Solid Edge part; units mm, degrees
sketch "Sketch1" plane through (0, 0, 0) normal (0, -1, 0) x (1, 0, 0)
  line L0 (0, 120) -> (0, 0)
  line L1 (0, 0) -> (100, 0)
  line L2 (100, 0) -> (100, 120)
  line L3 (100, 120) -> (0, 120)
extrude "Protrusion1" add sketch "Sketch1" against normal blind 150
hole "Hole1" at (25, 25, 120) direction (0, 0, -1) diameter 8.376 depth 35 start chamfer 1 start chamfer angle 45
hole "Hole2" at (25, 125, 120) direction (0, 0, -1) diameter 8.376 depth 35 start chamfer 1 start chamfer angle 45
hole "Hole3" at (75, 125, 120) direction (0, 0, -1) diameter 8.376 depth 35 start chamfer 1 start chamfer angle 45
hole "Hole4" at (75, 25, 120) direction (0, 0, -1) diameter 8.376 depth 35 start chamfer 1 start chamfer angle 45
hole "Hole5" at (25, 25, 0) direction (0, 0, 1) diameter 8.376 depth 35 start chamfer 1 start chamfer angle 45
hole "Hole6" at (75, 25, 0) direction (0, 0, 1) diameter 8.376 depth 35 start chamfer 1 start chamfer angle 45
hole "Hole7" at (75, 125, 0) direction (0, 0, 1) diameter 8.376 depth 35 start chamfer 1 start chamfer angle 45
hole "Hole8" at (25, 125, 0) direction (0, 0, 1) diameter 8.376 depth 35 start chamfer 1 start chamfer angle 45
hole "Achsenhalterung_Schubkarr" at (0, 75, 60) direction (1, 0, 0) diameter 20 end through all start chamfer 1 start chamfer angle 45 end chamfer 1 end chamfer angle 45
Design review of the part built by this model. Coordinates are the model's own, in mm. A direction names the side the tool comes from. Coordinates: 2 decimals unless noted, no trailing zeros. Order: outer loops, then holes, each group sorted by start corner. A loop starts at its lowest first (then second) coordinate and runs counter-clockwise, first axis right, second up.
Item 1: For line 1 (Y direction, x = 75, z = 12); line 2 (X direction, y = 25, z = 15.5); line 3 (Y direction, x = 57, z = 60), list the stretches that pass through material, from the lowest coordinate up.
Item 2: Take a section at D-D, the plane x = 87. Write out the cut boundary in (y, z).
Item 3: For pin 1 Ø4 at (x, y) = (23, 126) entering from -Z; pin 2 Ø2.5 at (x, y) = (76, 24) entering from +Z; pin 3 Ø4 at (x, y) = (26.5, 23) entering from +Z, all flat-tipped, find the tip position at first contact; note any pin that passes through.
Item 4: The part is to be moulded in two halves that separate along Y. For faces 1 (the flat face through (0, 74, 74)), 2 (the flat face through (75, 25, 85)), 3 (the flat face through (51, 0, 61)), say which applies: pulls with the +Y half, pulls with the -Y half, needs draft (parallel to the pull), parting line crosses it, or undercut.
Item 5: Take a section at A-A, the plane y = 75. Write out the cut boundary in (x, z), then the cut area to 4 significant figures.
Item 6: Take a section at C-C, the plane y = 125. Write out the cut boundary in (x, z), then the cut area to 3 significant figures.
Item 7: For faces 4 (the flat face through (49, 74, 0)), 5 (the flat face through (25, 125, 35)), 6 (the cylindrical face through (22.17, 28.087, 101.762)), list the 3-axis set-ups (+Z, -Z, +X, -X, +Y, -Y) from which the entire face can be reached by the end or side of a thin tool; tool diameter is ignored.
The answers:
1. line 1: y = 0 to 20.81, 29.19 to 120.81, 129.19 to 150
1. line 2: x = 0 to 20.81, 29.19 to 70.81, 79.19 to 100
1. line 3: y = 0 to 65, 85 to 150
2. outline: (0, 0) - (150, 0) - (150, 120) - (0, 120) - close; hole circle Ø20 at (75, 60)
3. pin 1: stops at z = 0.95
3. pin 2: stops at z = 85
3. pin 3: stops at z = 119.31
4. face 1: needs draft
4. face 2: undercut
4. face 3: pulls with the -Y half
5. outline: (0, 0) - (100, 0) - (100, 49) - (99, 50) - (1, 50) - (0, 49) - close; (0, 71) - (1, 70) - (99, 70) - (100, 71) - (100, 120) - (0, 120) - close
5. area: 10,000 mm2
6. outline: (0, 0) - (19.81, 0) - (20.81, 1) - (20.81, 35) - (29.19, 35) - (29.19, 1) - (30.19, 0) - (69.81, 0) - (70.81, 1) - (70.81, 35) - (79.19, 35) - (79.19, 1) - (80.19, 0) - (100, 0) - (100, 120) - (80.19, 120) - (79.19, 119) - (79.19, 85) - (70.81, 85) - (70.81, 119) - (69.81, 120) - (30.19, 120) - (29.19, 119) - (29.19, 85) - (20.81, 85) - (20.81, 119) - (19.81, 120) - (0, 120) - close
6. area: 10,800 mm2
7. face 4: -Z, +X, -X, +Y, -Y
7. face 5: -Z
7. face 6: +Z
